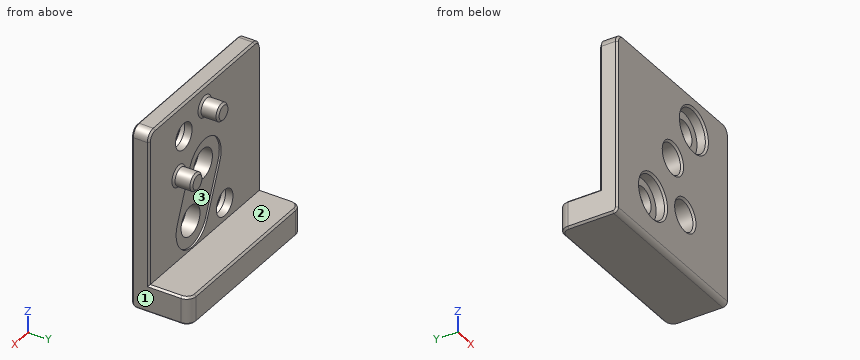
from build123d import *

# Parameters (mm, degrees)
SKETCH1_W           = 19.4
SKETCH1_H           = 1.9
SKETCH1_W_2         = 3
SKETCH1_H_2         = 4.4
BOSS_EXTRUDE1_DEPTH = 9.4
SKETCH2_R           = 1.6
SKETCH2_R_2         = 1.4
CUT_EXTRUDE1_DEPTH  = 23.001818107
CUT_EXTRUDE2_DEPTH  = 0.2
SKETCH4_R           = 2.25
CUT_EXTRUDE3_DEPTH  = 1.1
FILLET1_R           = 1
SKETCH5_R           = 0.95
BOSS_EXTRUDE2_DEPTH = 2
FILLET4_R           = 0.5
CHAMFER1_SIZE       = 0.2


with BuildPart() as part:
    # Sketch1 → Boss-Extrude1 (new, symmetric)
    with BuildSketch(Plane(origin=(0, 0, 0), x_dir=(0, 0, -1), z_dir=(1, 0, 0))):
        with Locations((9.7, -0.95)):
            Rectangle(SKETCH1_W, SKETCH1_H)
        with Locations((17.9, 2.2)):
            Rectangle(SKETCH1_W_2, SKETCH1_H_2)
    extrude(amount=BOSS_EXTRUDE1_DEPTH, both=True)

    # Sketch2 → Cut-Extrude1 (cut, through all)
    with BuildSketch(Plane(origin=(0, 0, 0), x_dir=(1, 0, 0), z_dir=(0, 1, 0))):
        with Locations(Location((0, 8.5, 0), (0, 0, 270))):
            Circle(SKETCH2_R)
        with Locations(Location((2.1, 13.5, 0), (0, 0, 270))):
            Circle(SKETCH2_R)
        with Locations(Location((3.55, 3.5, 0), (0, 0, 270))):
            Circle(SKETCH2_R_2)
        with Locations(Location((-3.35, 14.5, 0), (0, 0, 270))):
            Circle(SKETCH2_R_2)
    extrude(amount=-CUT_EXTRUDE1_DEPTH, mode=Mode.SUBTRACT)

    # Sketch3 → Cut-Extrude2 (cut)
    with BuildSketch(Plane(origin=(0, 0, 0), x_dir=(1, 0, 0), z_dir=(0, 1, 0))):
        with BuildLine():
            Line((-2.53545079, 9.564889332), (-0.43545079, 14.564889332))
            ThreePointArc((-0.43545079, 14.564889332), (3.164889332, 16.03545079), (4.63545079, 12.435110668))
            Line((4.63545079, 12.435110668), (2.53545079, 7.435110668))
            ThreePointArc((2.53545079, 7.435110668), (-1.064889332, 5.96454921), (-2.53545079, 9.564889332))
        make_face()
    extrude(amount=-CUT_EXTRUDE2_DEPTH, mode=Mode.SUBTRACT)

    # Sketch4 → Cut-Extrude3 (cut)
    with BuildSketch(Plane.XZ.offset(1.9)):
        with Locations(Location((-3.35, -14.5, 0), (0, 0, 270))):
            Circle(SKETCH4_R)
        with Locations(Location((3.55, -3.5, 0), (0, 0, 270))):
            Circle(SKETCH4_R)
    extrude(amount=-CUT_EXTRUDE3_DEPTH, mode=Mode.SUBTRACT)

    # Fillet1
    fillet1_edges = [part.edges().sort_by_distance(p)[0] for p in [
        (9.4, 4.4, -17.9),
        (9.4, -0.95, 0),
        (-9.4, -0.95, 0),
        (-9.4, 4.4, -17.9),
    ]]
    fillet(fillet1_edges, radius=FILLET1_R)

    # Sketch5 → Boss-Extrude2 (add)
    with BuildSketch(Plane(origin=(0, 0, 0), x_dir=(1, 0, 0), z_dir=(0, 1, 0))):
        with Locations(Location((0, 2.2, 0), (0, 0, 270))):
            Circle(SKETCH5_R)
        with Locations(Location((4.4, 7.3, 0), (0, 0, 270))):
            Circle(SKETCH5_R)
    extrude(amount=BOSS_EXTRUDE2_DEPTH)

    # Fillet4
    fillet4_edges = [part.edges().sort_by_distance(p)[0] for p in [
        (0, -1.9, -19.4),
    ]]
    fillet(fillet4_edges, radius=FILLET4_R)

    # Chamfer1
    chamfer1_edges = [part.edges().sort_by_distance(p)[0] for p in [
        (4.4, 0, -8.25),
        (4.4, 2, -8.25),
        (-9.4, -1.753553391, -19.253553391),
        (9.4, -1.753553391, -19.253553391),
        (9.4, 1.7, -16.4),
        (2.1, -1.9, -15.1),
        (0, -1.9, -10.1),
        (-3.35, -1.9, -12.25),
        (3.55, -1.9, -1.25),
        (0, 4.4, -16.4),
        (0, 4.4, -19.4),
        (9.107106781, 4.107106781, -16.4),
        (-9.107106781, 4.107106781, -16.4),
        (-9.4, 1, -19.4),
        (-9.4, -1.9, -9.95),
        (-9.4, 0, -8.7),
        (9.4, 1, -19.4),
        (9.107106781, 4.107106781, -19.4),
        (-9.107106781, 4.107106781, -19.4),
        (9.4, 0, -8.7),
        (9.4, -1.9, -9.95),
        (0, -1.9, 0),
        (0, 0, 0),
        (9.107106781, -1.9, -0.292893219),
        (-9.107106781, -1.9, -0.292893219),
        (9.107106781, 0, -0.292893219),
        (-9.107106781, 0, -0.292893219),
        (-9.4, 1.7, -16.4),
        (0, 0, -3.15),
        (0, 2, -3.15),
    ]]
    chamfer(chamfer1_edges, length=CHAMFER1_SIZE)


solid = part.part
For this review, take the finished solid that the model builds, in its own axes (mm). Face numbers are marked on the shaded views. Round coordinates to 2 decimals unless told otherwise and drop trailing zeros. Loops run counter-clockwise (first coordinate to the right, second up) from the corner with the lowest first, then second, coordinate; pieces in that order, holes last. Notation, with made-up numbers: (57, -20) - (97, -20) arc R10 ccw to (97, -9) - close; hole circle Ø11 at (17, -28.5). An arc over 180 degrees is marked (long way). One line per item, written item: value. Start each with the question number.
Item 1: Take a section at A-A (y = 1). Give the boundary of the cut face in (x, z), plus the area to 3 significant figures.
Item 2: For L1, parallel to X at y = -0.6, z = -8.5; L2, parallel to X at y = -1.45, z = -3.5; L3, parallel to X at y = -0.55, z = -13.5, list the stretches that pass through material, from the lowest coordinate up.
Item 3: Take a section at C-C (y = -0.5). Give the boundary of the cut face in (x, z).
Item 4: Take a section at B-B (x = -3.35). Give the boundary of the cut face in (y, z), plus the area to 3 significant figures.
Item 5: The part is to be moulded in two halves that separate along X. For the marked faces 1, 2 and 3, say which applies: +X half, -X half, draft (parallel to the pull), parting line (faces both ways), or undercut.
Item 6: Clearance check with flat-ended pins moving along their axes: pin 1 Ø4.5 at (x, z) = (3.55, -3.5) entering from +Y; pin 2 Ø1.7 at (x, z) = (-3.35, -14.5) entering from -Y; pin 3 Ø3.5 at (x, z) = (2.1, -13.5) entering from +Y; pin 4 Ø8 at (x, z) = (1, -7.5) entering from +Y. State where each tip first meets the part, or that it passes through.
Item 7: Take a section at D-D (x = -7.75). Give the boundary of the cut face in (y, z).
Answer below:
1. outline: (-9.4, -19.2) - (-9.2, -19.4) - (9.2, -19.4) - (9.4, -19.2) - (9.4, -16.6) - (9.2, -16.4) - (-9.2, -16.4) - (-9.4, -16.6) - close; circle Ø1.9 at (0, -2.2); circle Ø1.9 at (4.4, -7.3)
1. area: 62.0 mm2
2. L1: x = -9.4 to -1.6, 1.6 to 9.4
2. L2: x = -9.4 to 1.3, 5.8 to 9.4
2. L3: x = -9.4 to -4.33, -2.37 to 0.5, 3.7 to 9.4
3. outline: (-9.4, -19.2) - (-9.2, -19.4) - (9.2, -19.4) - (9.4, -19.2) - (9.4, -1) arc R1 ccw to (8.4, 0) - (-8.4, 0) arc R1 ccw to (-9.4, -1) - close; hole circle Ø2.8 at (-3.35, -14.5); hole circle Ø3.2 at (0, -8.5); hole circle Ø3.2 at (2.1, -13.5); hole circle Ø2.8 at (3.55, -3.5)
4. outline: (-1.9, -18.9) arc R0.5 ccw to (-1.4, -19.4) - (4.2, -19.4) - (4.4, -19.2) - (4.4, -16.6) - (4.2, -16.4) - (0, -16.4) - (0, -15.9) - (-0.8, -15.9) - (-0.8, -16.75) - (-1.7, -16.75) - (-1.9, -16.95) - close; (-1.9, -12.05) - (-1.7, -12.25) - (-0.8, -12.25) - (-0.8, -13.1) - (0, -13.1) - (0, -0.2) - (-0.2, 0) - (-1.7, 0) - (-1.9, -0.2) - close
4. area: 42.7 mm2
5. face 1: +X half
5. face 2: draft
5. face 3: undercut
6. pin 1: stops at y = 0
6. pin 2: passes through
6. pin 3: stops at y = -0.2
6. pin 4: stops at y = 2
7. outline: (-1.9, -18.9) arc R0.5 ccw to (-1.4, -19.4) - (4.2, -19.4) - (4.4, -19.2) - (4.4, -16.6) - (4.2, -16.4) - (0, -16.4) - (0, -0.2) - (-0.2, 0) - (-1.7, 0) - (-1.9, -0.2) - close
